Job drawing, mm, ordinate dimensions from the low corner. One solid piece. A direction names the side the tool comes from. Give positions to 0.01 mm unless a question says otherwise; leave off trailing zeros. Order: outer loops, then holes, each group sorted by start corner. A loop starts at its lowest first (then second) coordinate and runs counter-clockwise, first axis right, second up. Notation, with made-up numbers: (71.5, -32) - (119.5, -32) arc R21 ccw to (119.5, -27) - close; hole circle Ø8 at (76, 77). An arc over 180 degrees is marked (long way). Write each question's results on one line, items separated by ' | '. Start each with the question number.
1) Tool access for the marked faces 1 and 2: list every direction of +Z, -Z, +X, -X, +Y, -Y with a clear straight run to the whole face (end or side of a thin tool).
2) Drill centre lines: line 1 along X through (y, z) = (1.85, 13); line 2 along X through (y, z) = (6.25, 10); line 3 along Z through (x, y) = (9.25, 1) (1 decimal). Where is each one in solid material? Low to high. Write a range as from..to.
3) Cut at B-B on x = 10. List the corners of the cut face in (y, z).
4) Cut at D-D on z = 13. List the corners of the cut face in (x, y).
5) Drop flat-ended pins along their axis: pin 1 Ø2 at (x, y) = (5, 3) entering from +Z (1 decimal); pin 2 Ø3 at (y, z) = (1.5, 8) entering from +X; pin 3 Ø5 at (x, y) = (3.5, 1.5) entering from -Z (1 decimal). Give the stop position or say it passes through.
6) Cut at C-C on x = 8. List the corners of the cut face in (y, z).
7) Cut at A-A on z = 10. List the corners of the cut face in (x, y).
8) Two-plate mould, pull along Z, no slides. Class the marked faces 3, 4 and 5: +Z half, -Z half, draft (parallel to the pull), parting line (faces both ways), or undercut.
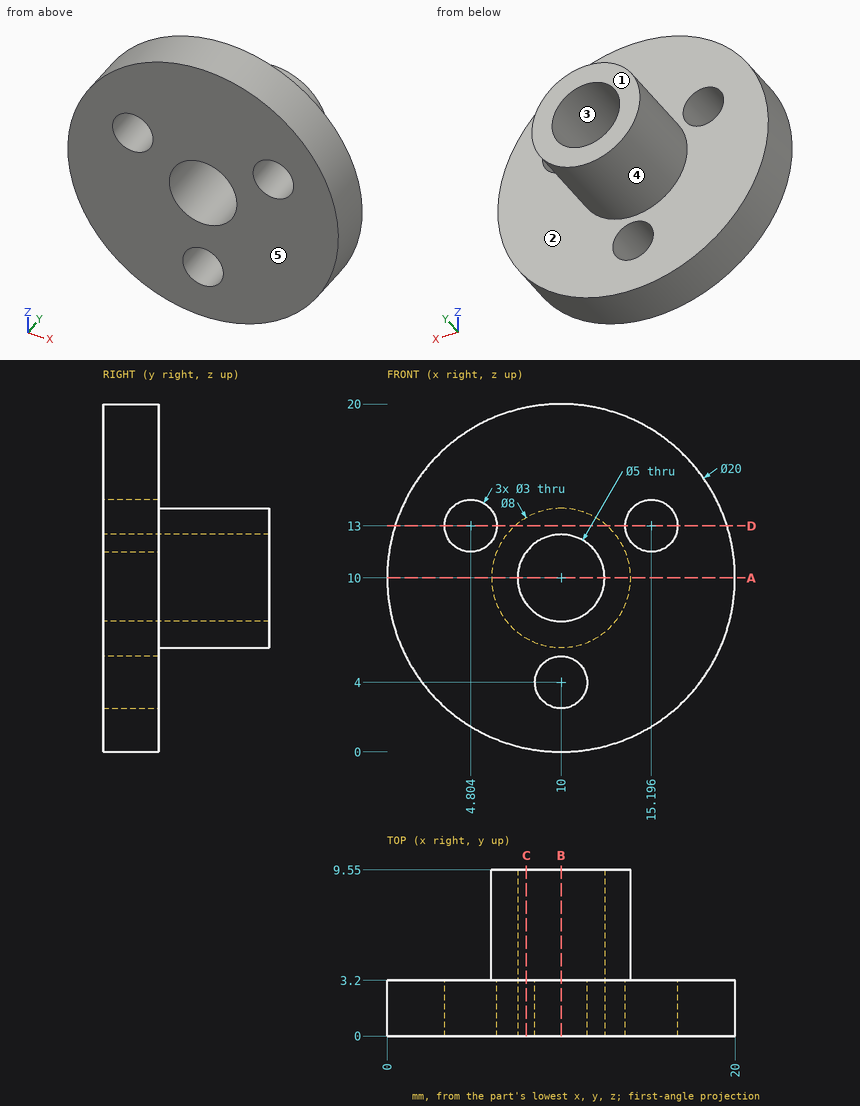
Results:
1) face 1: +Z, -Z, +X, -X, +Y | face 2: +Y
2) line 1: 0.46..3.3, 6.3..13.7, 16.7..19.54 | line 2: 6..7.5, 12.5..14 | line 3: 0..2.7, 5.3..7.6, 12.4..20
3) outline: (0, 0) - (3.2, 0) - (3.2, 2.5) - (0, 2.5) - close; (0, 5.5) - (3.2, 5.5) - (3.2, 6) - (9.55, 6) - (9.55, 7.5) - (0, 7.5) - close; (0, 12.5) - (9.55, 12.5) - (9.55, 14) - (3.2, 14) - (3.2, 20) - (0, 20) - close
4) outline: (0.46, 0) - (3.3, 0) - (3.3, 3.2) - (0.46, 3.2) - close; (6.3, 0) - (13.7, 0) - (13.7, 3.2) - (12.65, 3.2) - (12.65, 9.55) - (7.35, 9.55) - (7.35, 3.2) - (6.3, 3.2) - close; (16.7, 0) - (19.54, 0) - (19.54, 3.2) - (16.7, 3.2) - close
5) pin 1: z = 19.2 | pin 2: x = 19.99 | pin 3: z = 0.8
6) outline: (0, 0.2) - (3.2, 0.2) - (3.2, 6.54) - (9.55, 6.54) - (9.55, 8.5) - (0, 8.5) - close; (0, 11.5) - (9.55, 11.5) - (9.55, 13.46) - (3.2, 13.46) - (3.2, 19.8) - (0, 19.8) - close
7) outline: (0, 0) - (7.5, 0) - (7.5, 9.55) - (6, 9.55) - (6, 3.2) - (0, 3.2) - close; (12.5, 0) - (20, 0) - (20, 3.2) - (14, 3.2) - (14, 9.55) - (12.5, 9.55) - close
8) face 3: undercut | face 4: parting line | face 5: draft
